```python
from build123d import *

# Parameters (mm, degrees)
BOSS_EXTRUDE1_DEPTH = 3
SKETCH2_R           = 14.75
BOSS_EXTRUDE2_DEPTH = 3
SKETCH5_R           = 15.25
SKETCH5_R_2         = 14.75
BOSS_EXTRUDE3_DEPTH = 3


with BuildPart() as part:
    # Sketch1 → Boss-Extrude1 (new body)
    with BuildSketch(Plane.XY):
        with BuildLine():
            ThreePointArc((0, 30), (21.984686874, 11.144587301), (24.197417864, -17.733724051))
            ThreePointArc((24.197417864, -17.733724051), (-1.457844914, -26.759103366), (-25.980762114, -15))
            ThreePointArc((-25.980762114, -15), (-22.31018621, 12.880792014), (0, 30))
        make_face()
    extrude(amount=BOSS_EXTRUDE1_DEPTH)

    # Sketch2 → Boss-Extrude2 (add)
    with BuildSketch(Plane.XY.offset(3)):
        with Locations(Location((0, 30, 0), (0, 0, 206.579187248))):
            Circle(SKETCH2_R)
        with Locations(Location((24.197417864, -17.733724051, 0), (0, 0, 209.902892112))):
            Circle(SKETCH2_R)
        with Locations(Location((-25.980762114, -15, 0), (0, 0, 93.420812752))):
            Circle(SKETCH2_R)
    extrude(amount=BOSS_EXTRUDE2_DEPTH)

    # Sketch5 → Boss-Extrude3 (add)
    with BuildSketch(Plane(origin=(0, 0, 0), x_dir=(-1, 0, 0), z_dir=(0, 0, -1))):
        with Locations(Location((0, 0, 0), (0, 0, 180))):
            Circle(SKETCH5_R)
        Circle(SKETCH5_R_2, mode=Mode.SUBTRACT)
    extrude(amount=BOSS_EXTRUDE3_DEPTH)


solid = part.part
```
Build history of the part. All positions in model axes, mm. A direction names the side the tool comes from. Round coordinates to 2 decimals unless told otherwise and drop trailing zeros. Write each loop counter-clockwise with the first axis right and the second up, starting at its lowest first coordinate (ties: lowest second). Pieces come first, ordered by that corner, then holes.
1) 3-axis set-ups, long thin cutter, end or side, ignore diameter. For faces 1 (the cylindrical face through (37.295, -10.95, 4.479)), 2 (the flat face through (-12, -11, 0)), 3 (the cylindrical face through (21.8, 11.5, 1.5)): which of +Z, -Z, +X, -X, +Y, -Y reach the whole face in a straight line?
2) Band-saw the part on C-C, the plane z = -2. List the corners of the cut face in (x, y), and give its area (3 significant figures).
3) Mould opens along Y. For faces 4 (the flat face through (-1, -15, -3)), 5 (the cylindrical face through (-3.58, 44.31, 4.48)), 6 (the cylindrical face through (-3.306, 14.887, -1.479)), 7 (the cylindrical face through (-1.07, -26.78, 1.48)) say: +Y half, -Y half, draft (parallel to the pull), parting line (faces both ways), or undercut.
4) Pin check, flat tips, straight feed: pin 1 (12 mm diameter, centred on x = -13.5, y = 2, fed in from +Z); pin 2 (3 mm diameter, centred on y = 32.5, z = 3.5, fed in from -X); pin 3 (6.5 mm diameter, centred on x = 3, y = 38, fed in from -Z); pin 4 (16 mm diameter, centred on x = 3, y = 8.5, fed in from -Z). Stop position of each tip, or through.
5) Band-saw the part on A-A, the plane y = -10. List the corners of the cut face in (x, z).
6) Drill centre lines: probe 1 along Y at (x, z) = (0, -1); probe 2 along Z at (x, y) = (-10.5, 24.5); probe 3 along Z at (x, y) = (-33.5, -15.5). Where is each one in solid material? Low to high.
7) Band-saw the part on D-D, the plane z = 4.5. List the corners of the cut face in (x, y).
8) Band-saw the part on B-B, the plane x = 1. List the corners of the cut face in (y, z).
Ans:
1. face 1: +Z
1. face 2: -Z
1. face 3: -Z, +X
2. outline: circle Ø30.5 at (0, 0); hole circle Ø29.5 at (0, 0)
2. area: 47.1 mm2
3. face 4: draft
3. face 5: undercut
3. face 6: parting line
3. face 7: -Y half
4. pin 1: stops at z = 3
4. pin 2: stops at x = -14.72
4. pin 3: stops at z = 3
4. pin 4: stops at z = -3
5. outline: (-39.86, 3) - (-26.95, 3) - (-26.95, 0) - (-11.51, 0) - (-11.51, -3) - (-10.84, -3) - (-10.84, 0) - (10.84, 0) - (10.84, -3) - (11.51, -3) - (11.51, 0) - (25.86, 0) - (25.86, 3) - (36.76, 3) - (36.76, 6) - (11.64, 6) - (11.64, 3) - (-12.1, 3) - (-12.1, 6) - (-39.86, 6) - close
6. probe 1: y = -15.25 to -14.75, 14.75 to 15.25
6. probe 2: z = 0 to 6
6. probe 3: z = 3 to 6
7. outline: circle Ø29.5 at (-25.98, -15); circle Ø29.5 at (0, 30); circle Ø29.5 at (24.2, -17.73)
8. outline: (-26.81, 0) - (-15.22, 0) - (-15.22, -3) - (-14.72, -3) - (-14.72, 0) - (14.72, 0) - (14.72, -3) - (15.22, -3) - (15.22, 0) - (29.66, 0) - (29.66, 3) - (44.72, 3) - (44.72, 6) - (15.28, 6) - (15.28, 3) - (-26.81, 3) - close
